Model file for the job. Use its own axes, mm. Face numbers are marked on the shaded views. A direction names the side the tool comes from. Round coordinates to 2 decimals unless told otherwise and drop trailing zeros. Write each loop counter-clockwise with the first axis right and the second up, starting at its lowest first coordinate (ties: lowest second). Pieces come first, ordered by that corner, then holes. Notation, with made-up numbers: (68, 38) - (90, 38) arc R15 ccw to (90, 53) - close; hole circle Ø8 at (16.25, 61). An arc over 180 degrees is marked (long way). One line per item, written item: value.
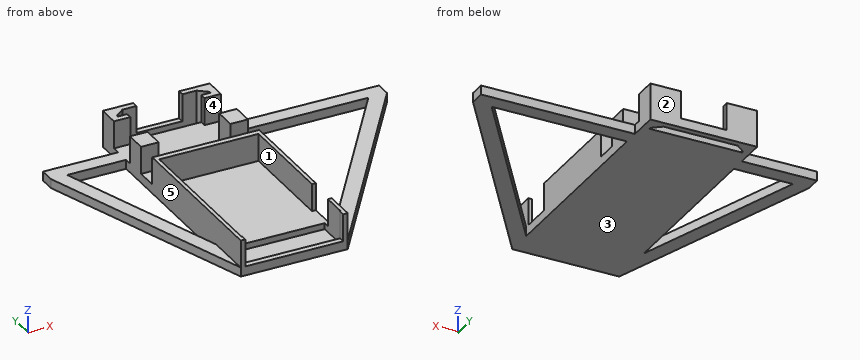
from build123d import *

# Parameters (mm, degrees)
F0_W     = 5
F0_H     = 5
F0_W_2   = 5.75
F0_H_2   = 7
F1_DEPTH = 3
F2_DEPTH = 1
F3_DEPTH = 12


# Not quite as in the source:
# - a feature names something its author has since deleted; it is built from what else it names


with BuildPart() as f1:
    # F0 (on Top) → F1 (new body)
    with BuildSketch(Plane.XY):
        Polygon((-7.5, 41.25), (-7.5, 43.25), (-17.5, 43.25), (-17.5, 36.25), (-12.15, 36.25), (-12.15, 38.25), (-15.15, 38.25), (-15.15, 38.85), (-12.15, 41.25), align=None)
        Polygon((7.5, 43.25), (0, 43.25), (-7.5, 43.25), (-7.5, 41.25), (0, 41.25), (7.5, 41.25), align=None)
        Polygon((17.5, 43.25), (7.5, 43.25), (7.5, 41.25), (12.15, 41.25), (15.15, 38.85), (15.15, 38.25), (12.15, 38.25), (12.15, 36.25), (17.5, 36.25), align=None)
        Polygon((-17.5, 0), (-17.5, -27.8208897438), (-17.5, -43.25), (-16, -43.25), (-16, -41.25), (-16.25, -41.25), (-16.25, -31.25), (-16.25, 10.25), (0, 10.25), (16.25, 10.25), (16.25, -23.25), (17.5, -23.25), (17.5, 0), (17.5, 12.25), (-17.5, 12.25), align=None)
        Polygon((16.25, -33.25), (17.5, -33.25), (17.5, -23.25), (16.25, -23.25), (16.25, -31.25), align=None)
        Polygon((62.8901566565, 28.5934534669), (61.7828955537, 28.5934534669), (17.5, -34.5426103437), (17.5, -43.25), (67.8901566565, 28.5934534669), align=None)
        Polygon((-17.5, 28.5934534669), (-17.5, 33.5934534669), (-37.1098433435, 33.5934534669), (-37.1098433435, 28.5934534669), (-36.8246298966, 28.5934534669), align=None)
        with Locations((-39.6098433435, 31.0934534669)):
            Rectangle(F0_W, F0_H)
        with Locations((65.3901566565, 31.0934534669)):
            Rectangle(F0_W, F0_H)
        Polygon((62.8901566565, 33.5934534669), (17.5, 33.5934534669), (17.5, 28.5934534669), (61.7828955537, 28.5934534669), (62.8901566565, 28.5934534669), align=None)
        Polygon((16.25, -31.25), (16.25, -23.25), (16.25, 10.25), (0, 10.25), (-16.25, 10.25), (-16.25, -31.25), align=None)
        Polygon((-17.5, -27.8208897438), (-36.8246298966, 28.5934534669), (-37.1098433435, 28.5934534669), (-42.1098433435, 28.5934534669), (-17.5, -43.25), align=None)
        Polygon((-16, -41.25), (-16, -43.25), (0, -43.25), (16, -43.25), (16, -41.25), (0, -41.25), align=None)
        Polygon((17.5, -43.25), (17.5, -34.5426103437), (17.5, -33.25), (16.25, -33.25), (16.25, -41.25), (16, -41.25), (16, -43.25), align=None)
        Polygon((-12.15, 36.25), (-17.5, 36.25), (-17.5, 33.5934534669), (-17.5, 28.5934534669), (-17.5, 26.25), (-11.75, 26.25), (-11.75, 19.25), (-17.5, 19.25), (-17.5, 12.25), (17.5, 12.25), (17.5, 19.25), (11.75, 19.25), (11.75, 26.25), (17.5, 26.25), (17.5, 28.5934534669), (17.5, 33.5934534669), (17.5, 36.25), (12.15, 36.25), (12.15, 38.25), (0, 38.25), (-12.15, 38.25), align=None)
        with Locations((-14.625, 22.75)):
            Rectangle(F0_W_2, F0_H_2)
        with Locations((14.625, 22.75)):
            Rectangle(F0_W_2, F0_H_2)
    extrude(amount=F1_DEPTH)

    # F0 (on Top) → F2 (join)
    with BuildSketch(Plane.XY):
        Polygon((16.25, -41.25), (16.25, -33.25), (16.25, -31.25), (-16.25, -31.25), (-16.25, -41.25), (-16, -41.25), (0, -41.25), (16, -41.25), align=None)
    extrude(amount=F2_DEPTH)

    # F0 (on Top) → F3 (join)
    with BuildSketch(Plane.XY):
        Polygon((-7.5, 41.25), (-7.5, 43.25), (-17.5, 43.25), (-17.5, 36.25), (-12.15, 36.25), (-12.15, 38.25), (-15.15, 38.25), (-15.15, 38.85), (-12.15, 41.25), align=None)
        Polygon((17.5, 43.25), (7.5, 43.25), (7.5, 41.25), (12.15, 41.25), (15.15, 38.85), (15.15, 38.25), (12.15, 38.25), (12.15, 36.25), (17.5, 36.25), align=None)
        Polygon((-17.5, 0), (-17.5, -27.8208897438), (-17.5, -43.25), (-16, -43.25), (-16, -41.25), (-16.25, -41.25), (-16.25, -31.25), (-16.25, 10.25), (0, 10.25), (16.25, 10.25), (16.25, -23.25), (17.5, -23.25), (17.5, 0), (17.5, 12.25), (-17.5, 12.25), align=None)
        Polygon((17.5, -43.25), (17.5, -34.5426103437), (17.5, -33.25), (16.25, -33.25), (16.25, -41.25), (16, -41.25), (16, -43.25), align=None)
        with Locations((-14.625, 22.75)):
            Rectangle(F0_W_2, F0_H_2)
        with Locations((14.625, 22.75)):
            Rectangle(F0_W_2, F0_H_2)
    extrude(amount=F3_DEPTH)


solid = f1.part
1. Mould opens along Y. For the marked faces 1, 2 and 3 say: released by +Y, released by -Y, zero draft, split by the parting line, or undercut.
Report:
face 1: undercut
face 2: released by +Y
face 3: zero draft
2. Tool access for the marked faces 4 and 5: list every direction of +Z, -Z, +X, -X, +Y, -Y with a clear straight run to the whole face (end or side of a thin tool).
Report:
face 4: +Z, +X, -X
face 5: +Z
3. Band-saw the part on A-A on y = -25.5. Write the cut outline in (x, z), plus the area to 3 significant figures.
Report:
outline: (-23.58, 0) - (-18.3, 0) - (-18.3, 3) - (-23.58, 3) - close; (-17.5, 0) - (17.5, 0) - (17.5, 3) - (-16.25, 3) - (-16.25, 12) - (-17.5, 12) - close; (23.84, 0) - (29.95, 0) - (29.95, 3) - (23.84, 3) - close
area: 150 mm²
4. Band-saw the part on B-B on x = -19. Write the cut outline in (y, z).
Report:
outline: (-38.87, 0) - (-23.44, 0) - (-23.44, 3) - (-38.87, 3) - close; (28.59, 0) - (33.59, 0) - (33.59, 3) - (28.59, 3) - close
5. Band-saw the part on D-D on x = 45. Write the cut outline in (y, z).
Report:
outline: (-4.04, 0) - (4.67, 0) - (4.67, 3) - (-4.04, 3) - close; (28.59, 0) - (33.59, 0) - (33.59, 3) - (28.59, 3) - close
6. Band-saw the part on C-C on z = 9. State how many separate pieces and enclosed holes the cut face has, plus the area to 3 significant figures.
Report:
separate pieces: 6
enclosed holes: 0
area: 355 mm²
7. Wall check: probe 1 along Y at (x, z) = (1, 2.25); probe 2 along Y at (x, z) = (7, 0.5); probe 3 along X at (y, z) = (24, 9.5). Give the ranges that are in metal, low to high. Write a range as [from, to].
Report:
probe 1: [-43.25, -41.25], [-31.25, 38.25], [41.25, 43.25]
probe 2: [-43.25, 38.25], [41.25, 43.25]
probe 3: [-17.5, -11.75], [11.75, 17.5]
8. Drop flat-ended pins along their axis: pin 1 (8 mm diameter, centred on x = -29.5, y = 21, fed in from +Z); pin 2 (0.5 mm diameter, centred on y = 38.5, z = 8.5, fed in from +X); pin 3 (8 mm diameter, centred on x = 4.5, y = -38, fed in from +Z); pin 4 (7 mm diameter, centred on x = -4, z = 6, fed in from +Y). Give the stop position or say it passes through.
Report:
pin 1: through
pin 2: x = 17.5
pin 3: z = 3
pin 4: y = 43.25
